from build123d import *

# Parameters (mm, degrees)
PRISM001_DEPTH    = 6.5
FILLET018_R       = 0.3
CYLINDER012_R     = 1.5
CYLINDER012_DEPTH = 3.4
CYLINDER013_R     = 1
CYLINDER013_DEPTH = 6.5


with BuildPart() as part:
    # Prism001 → Prism001 (join)
    with BuildSketch(Plane(origin=(12.5, 25.5, 6.3), x_dir=(0, 0, -1), z_dir=(0, -1, 0))):
        Polygon((2, 0), (1, 1.732051), (-1, 1.732051), (-2, 0), (-1, -1.732051), (1, -1.732051), align=None)
    extrude(amount=PRISM001_DEPTH)

    # Fillet018
    fillet018_edges = [part.edges().sort_by_distance(p)[0] for p in [
        (12.5, 22.25, 8.3),
        (14.232051, 22.25, 7.3),
        (10.767949, 22.25, 7.3),
        (14.232051, 22.25, 5.3),
        (12.5, 22.25, 4.3),
        (10.767949, 22.25, 5.3),
    ]]
    fillet(fillet018_edges, radius=FILLET018_R)

    # Cylinder012 → Cylinder012 (join)
    with BuildSketch(Plane(origin=(12.5, 19, 6.3), x_dir=(1, 0, 0), z_dir=(0, -1, 0))):
        Circle(CYLINDER012_R)
    extrude(amount=CYLINDER012_DEPTH)

    # Cylinder013 → Cylinder013 (cut)
    with BuildSketch(Plane(origin=(12.5, 26, 6.3), x_dir=(1, 0, 0), z_dir=(0, -1, 0))):
        Circle(CYLINDER013_R)
    extrude(amount=CYLINDER013_DEPTH, mode=Mode.SUBTRACT)


with BuildPart() as part_1:
    # Body007 placement: moved
    add(part.part.moved(Location((-25, 0, 0))))


solid = part_1.part
Design review of the part built by this model. Coordinates are the model's own, in mm. A direction names the side the tool comes from. Coordinates: 2 decimals unless noted, no trailing zeros. Loops run counter-clockwise (first coordinate to the right, second up) from the corner with the lowest first, then second, coordinate; pieces in that order, holes last. Notation, with made-up numbers: (71, 47.5) -> (81, 47.5) arc R14 ccw to (81, 56.5) -> close; hole circle Ø11 at (1, -37.75). An arc over 180 degrees is marked (long way). Use a Markdown table: item, result. Add a question column.
Item 1: We need section A-A, the plane z = 6.3. Write out the cut boundary in (x, y).
Item 2: Machinability: for faces 5 (the flat face through (-13.38, 22.3, 4.81)), 6 (the flat face through (-14, 19, 7)), which of the approach directions +Z, -Z, +X, -X, +Y, -Y give a long, thin tool a straight path to every point of the face, cutting with its end or side? Answer none if there is none.
Item 3: The part is to be moulded in two halves that separate along Z. For faces 1 (the cylindrical face through (-13.237, 22.542, 6.976)), 2 (the cylindrical face through (-12.695, 17.324, 7.787)), 3 (the flat face through (-13, 19.5, 6)), 4 (the flat face through (-10.768, 22, 6)), say which applies: +Z half, -Z half, draft (parallel to the pull), parting line (faces both ways), or undercut.
Item 4: We need section C-C, the plane x = -11.3. Write out the cut boundary in (y, z), and give its area (3 significant figures).
Item 5: We need section B-B, the plane x = -12.5. Write out the cut boundary in (y, z), and give its area (3 significant figures).
Item 6: We need section D-D, the plane z = 8. Write out the cut boundary in (x, y), and give its area (4 significant figures).
Item 7: Wall thickness on L1, parallel to X at y = 22.8, z = 6.3; L2, parallel to Z at x = -12.5, y = 23.45; L3, parallel to Y at x = -11.55, z = 6.2: over which ranges is each line inside the solid? List them lowest first. Write a range as from..to.
Numbers:
| question | item | result |
|---|---|---|
| 1 | outline | (-14.23, 19) -> (-14, 19) -> (-14, 15.6) -> (-11, 15.6) -> (-11, 19) -> (-10.77, 19) -> (-10.77, 25.5) -> (-11.5, 25.5) -> (-11.5, 19.5) -> (-13.5, 19.5) -> (-13.5, 25.5) -> (-14.23, 25.5) -> close |
| 2 | face 5 | -Z, -X, +Y, -Y |
| 2 | face 6 | -Y |
| 3 | face 1 | undercut |
| 3 | face 2 | parting line |
| 3 | face 3 | undercut |
| 3 | face 4 | draft |
| 4 | outline | (15.6, 5.4) -> (19, 5.4) -> (19, 4.99) -> (25.5, 4.99) -> (25.5, 7.61) -> (19, 7.61) -> (19, 7.2) -> (15.6, 7.2) -> close |
| 4 | area | 23.1 mm^2 |
| 5 | outline | (15.6, 4.8) -> (19, 4.8) -> (19, 4.35) -> (25.5, 4.35) -> (25.5, 5.3) -> (19.5, 5.3) -> (19.5, 7.3) -> (25.5, 7.3) -> (25.5, 8.25) -> (19, 8.25) -> (19, 7.8) -> (15.6, 7.8) -> close |
| 5 | area | 23.6 mm^2 |
| 6 | outline | (-13.02, 19) -> (-11.98, 19) -> (-11.98, 25.5) -> (-13.02, 25.5) -> close |
| 6 | area | 6.755 mm^2 |
| 7 | L1 | x = -14.23..-13.5, -11.5..-10.77 |
| 7 | L2 | z = 4.35..5.3, 7.3..8.25 |
| 7 | L3 | y = 15.6..19.5 |
